Autodesk Inventor part; units mm, degrees
ref_plane "YZ Plane" through (0, 0, 0) normal (1, 0, 0) x (0, 1, 0)
ref_plane "XZ Plane" through (0, 0, 0) normal (0, 1, 0) x (-1, 0, 0)
ref_plane "XY Plane" through (0, 0, 0) normal (0, 0, 1) x (1, 0, 0)
sketch "スケッチ1" plane through (0, 0, 0) normal (0, 0, 1) x (1, 0, 0)
  line L0 (32.5, 43.5) -> (-32.5, 43.5)
  line L1 (-32.5, 43.5) -> (-32.5, -43.5)
  line L2 (-32.5, -43.5) -> (32.5, -43.5)
  line L3 (32.5, -43.5) -> (32.5, 43.5)
  line L4 (32.5, 43.5) -> (-32.5, -43.5) construction
  line L5 (-32.5, 43.5) -> (32.5, -43.5) construction
  line L6 (-32.5, 29.7) -> (-11.7, 29.7)
  line L7 (-11.7, 29.7) -> (-11.7, -4.5)
  line L8 (-11.7, -4.5) -> (-32.5, -4.5)
  line L9 (-9.3, -43.5) -> (-9.3, -36.5)
  line L10 (-9.3, -36.5) -> (13.5, -36.5)
  line L11 (13.5, -36.5) -> (13.5, -43.5)
  line L12 (-29.7, -40.6) -> (16.7, -40.6) construction
  line L13 (16.7, -40.6) -> (16.7, 40.6) construction
  line L14 (16.7, 40.6) -> (-29.7, 40.6) construction
  line L15 (-29.7, 40.6) -> (-29.7, -40.6) construction
  line L16 (-29.7, -40.6) -> (16.7, 40.6) construction
  line L17 (16.7, -40.6) -> (-29.7, 40.6) construction
  circle A0 centre (16.7, 40.6) radius 1.6
  circle A1 centre (-29.7, 40.6) radius 1.6
  circle A2 centre (-29.7, -40.6) radius 1.6
  circle A3 centre (16.7, -40.6) radius 1.6
  line L18 (-32.5, 0) -> (32.5, 0) construction
  point P0 (0, 0)
  point P1 (0, 0)
  point P2 (0, 0)
  point P3 (-6.5, 0)
  dimension "d0" = 87
  dimension "d1" = 65
  dimension "d2" = 13.8
  dimension "d3" = 39
  dimension "d4" = 20.8
  dimension "d5" = 7
  dimension "d6" = 19
  dimension "d7" = 23.2
  dimension "d8" = 22.8
  dimension "d9" = 34.2
  dimension "d10" = 3.2
  dimension "d12" = 81.2
  dimension "d13" = 46.4
  dimension "d19" = 2.8
extrude "押し出し1" add sketch "スケッチ1" along normal blind 1.6 contours L3 L2 L11 L10 L9 L1 L8 L7 L6 L0
chamfer "面取り1" distance 1 angle 45 4 edges at (32.5, -43.5, 0.8) (-32.5, -43.5, 0.8) (32.5, 43.5, 0.8) (-32.5, 43.5, 0.8)
properties part number "A203-V2-Expansion-Board"
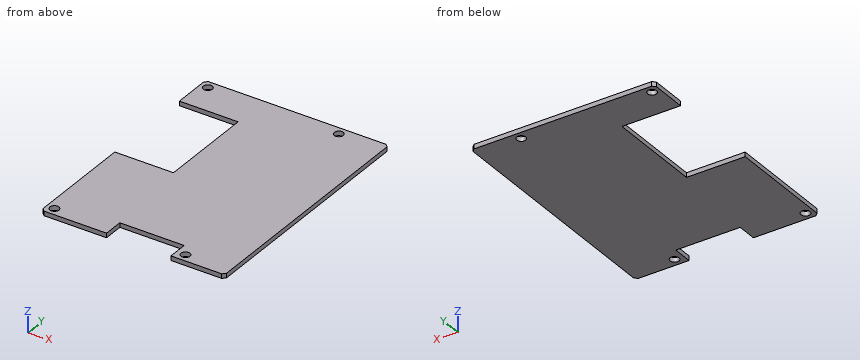
Part model, mm, in its own coordinate system. Give positions to 0.01 mm unless a question says otherwise; leave off trailing zeros. Loops run counter-clockwise (first coordinate to the right, second up) from the corner with the lowest first, then second, coordinate; pieces in that order, holes last.
(1) Band-saw the part on A-A (x = -25.5). Write the cut outline in (y, z).
Return value:
outline: (-43.5, 0) - (-4.5, 0) - (-4.5, 1.6) - (-43.5, 1.6) - close; (29.7, 0) - (43.5, 0) - (43.5, 1.6) - (29.7, 1.6) - close
(2) Band-saw the part on D-D (z = 0.25). Write the cut outline in (x, y).
Return value:
outline: (-32.5, -42.5) - (-31.5, -43.5) - (-9.3, -43.5) - (-9.3, -36.5) - (13.5, -36.5) - (13.5, -43.5) - (31.5, -43.5) - (32.5, -42.5) - (32.5, 42.5) - (31.5, 43.5) - (-31.5, 43.5) - (-32.5, 42.5) - (-32.5, 29.7) - (-11.7, 29.7) - (-11.7, -4.5) - (-32.5, -4.5) - close; hole circle Ø3.2 at (-29.7, -40.6); hole circle Ø3.2 at (-29.7, 40.6); hole circle Ø3.2 at (16.7, -40.6); hole circle Ø3.2 at (16.7, 40.6)
(3) Band-saw the part on B-B (y = -40.6). Write the cut outline in (x, z), and give its area (3 significant figures).
Return value:
outline: (-32.5, 0) - (-31.3, 0) - (-31.3, 1.6) - (-32.5, 1.6) - close; (-28.1, 0) - (-9.3, 0) - (-9.3, 1.6) - (-28.1, 1.6) - close; (13.5, 0) - (15.1, 0) - (15.1, 1.6) - (13.5, 1.6) - close; (18.3, 0) - (32.5, 0) - (32.5, 1.6) - (18.3, 1.6) - close
area: 57.3 mm2
(4) Band-saw the part on C-C (y = 40.6). Write the cut outline in (x, z), and give its area (3 significant figures).
Return value:
outline: (-32.5, 0) - (-31.3, 0) - (-31.3, 1.6) - (-32.5, 1.6) - close; (-28.1, 0) - (15.1, 0) - (15.1, 1.6) - (-28.1, 1.6) - close; (18.3, 0) - (32.5, 0) - (32.5, 1.6) - (18.3, 1.6) - close
area: 93.8 mm2
(5) Drill centre lines: line 1 along Y through (x, z) = (-29.7, 1.1); line 2 along Y through (x, z) = (16.7, 0.65); line 3 along X through (y, z) = (29, 1.5). Where is each one in solid material? Low to high.
Return value:
line 1: y = -43.5 to -42.2, -39 to -4.5, 29.7 to 39, 42.2 to 43.5
line 2: y = -43.5 to -42.2, -39 to 39, 42.2 to 43.5
line 3: x = -11.7 to 32.5
(6) Pin check, flat tips, straight feed: pin 1 (3.5 mm diameter, centred on x = -29.7, y = -40.6, fed in from -Z); pin 2 (0.8 mm diameter, centred on x = 7.5, z = 0.5, fed in from -Y); pin 3 (0.5 mm diameter, centred on y = 8.5, z = 0.5, fed in from -X). Stop position of each tip, or through.
Return value:
pin 1: stops at z = 0
pin 2: stops at y = -36.5
pin 3: stops at x = -11.7
